from build123d import *

# Parameters (mm, degrees)
SKETCH2_W           = 25.4
SKETCH2_H           = 19.05
BOSS_EXTRUDE1_DEPTH = 1.27
SKETCH3_R           = 3.81
BOSS_EXTRUDE2_DEPTH = 7.62
SKETCH4_R           = 2.54
CUT_EXTRUDE1_DEPTH  = 7.366


with BuildPart() as part:
    # Sketch2 → Boss-Extrude1 (new body)
    with BuildSketch(Plane.XY):
        with Locations((12.7, -9.525)):
            Rectangle(SKETCH2_W, SKETCH2_H)
    extrude(amount=BOSS_EXTRUDE1_DEPTH)

    # Sketch3 → Boss-Extrude2 (add)
    with BuildSketch(Plane.XY.offset(1.27)):
        with Locations(Location((12.7, -9.733398963, 0), (0, 0, 180))):
            Circle(SKETCH3_R)
    extrude(amount=BOSS_EXTRUDE2_DEPTH)

    # Sketch4 → Cut-Extrude1 (cut)
    with BuildSketch(Plane.XY.offset(8.89)):
        with Locations((12.7, -9.733398963)):
            Circle(SKETCH4_R)
    extrude(amount=-CUT_EXTRUDE1_DEPTH, mode=Mode.SUBTRACT)


solid = part.part
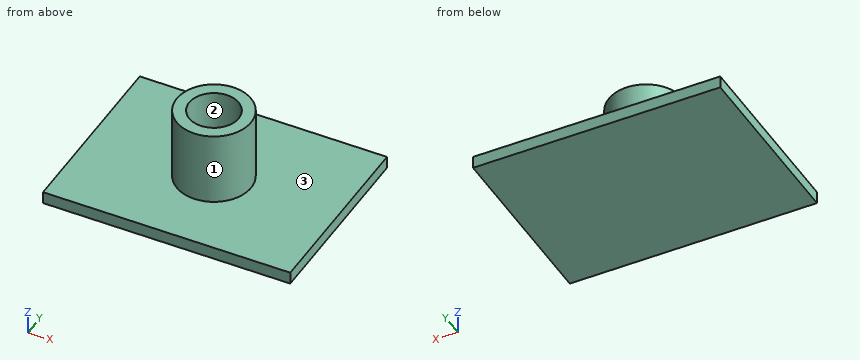
CAD build for the part. Positions are in the model's coordinates, mm. Face numbers are marked on the shaded views. Give positions to 0.01 mm unless a question says otherwise; leave off trailing zeros. Loops run counter-clockwise (first coordinate to the right, second up) from the corner with the lowest first, then second, coordinate; pieces in that order, holes last. Notation, with made-up numbers: M 89.25,63.5 L 112.25,63.5 A14 ccw 112.25,81.5 Z; hole C 3.5,87.5 d5. An arc over 180 degrees is marked long. Answer in a Markdown table with one row per item. Add a question column.
Item 1: Mould opens along Y. For the marked faces 1, 2 and 3 say: +Y half, -Y half, draft (parallel to the pull), parting line (faces both ways), or undercut.
Item 2: Band-saw the part on B-B on y = -11.25. Give the cut face in (x, z), then the cut area to 3 significant figures.
Item 3: Band-saw the part on D-D on y = -17. Give the cut face in (x, z), then the cut area to 3 significant figures.
Item 4: Band-saw the part on A-A on x = 12.7. Give the cut face in (y, z).
Item 5: Band-saw the part on C-C on z = 4.75. Give the cut face in (x, y).
Item 6: Drop flat-ended pins along their axis: P1, Ø1.5, axis at x = 13.5, y = -10, coming from the +Z side; P2, Ø5, axis at x = 16.5, y = -2.5, coming from the +Z side. Give the stop position or say it passes through.
Item 7: Probe probe 1 along Y at (x, z) = (12.7, 4); probe 2 along Z at (x, y) = (20.75, -16.75); probe 3 along Z at (x, y) = (12, -12). List the from-to ranges inside material, lowest first.
Reply:
| question | item | result |
|---|---|---|
| 1 | face 1 | parting line |
| 1 | face 2 | undercut |
| 1 | face 3 | draft |
| 2 | outline | M 0,0 L 25.4,0 L 25.4,1.27 L 16.2,1.27 L 16.2,8.89 L 14.74,8.89 L 14.74,1.52 L 10.66,1.52 L 10.66,8.89 L 9.2,8.89 L 9.2,1.27 L 0,1.27 Z |
| 2 | area | 55.5 mm^2 |
| 3 | outline | M 0,0 L 25.4,0 L 25.4,1.27 L 0,1.27 Z |
| 3 | area | 32.3 mm^2 |
| 4 | outline | M -19.05,0 L 0,0 L 0,1.27 L -5.92,1.27 L -5.92,8.89 L -7.19,8.89 L -7.19,1.52 L -12.27,1.52 L -12.27,8.89 L -13.54,8.89 L -13.54,1.27 L -19.05,1.27 Z |
| 5 | outline | C 12.7,-9.73 d7.62; hole C 12.7,-9.73 d5.08 |
| 6 | P1 | stops at z = 1.52 |
| 6 | P2 | stops at z = 1.27 |
| 7 | probe 1 | y = -13.54 to -12.27, -7.19 to -5.92 |
| 7 | probe 2 | z = 0 to 1.27 |
| 7 | probe 3 | z = 0 to 1.52 |
